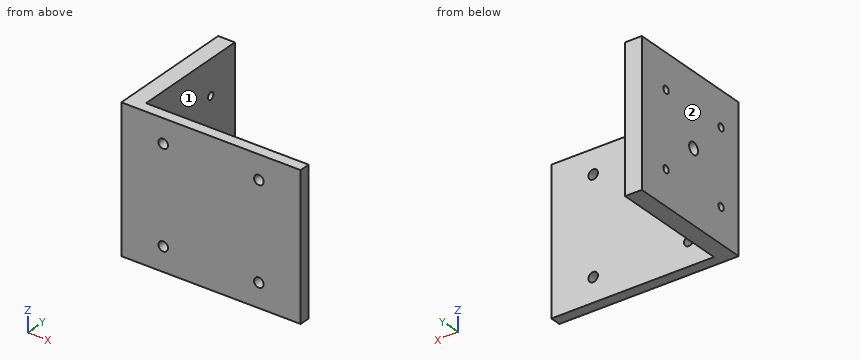
```python
from build123d import *

# Parameters (mm, degrees)
SKETCH1_W           = 75
SKETCH1_H           = 60
BOSS_EXTRUDE1_DEPTH = 4.5
SKETCH2_W           = 7
SKETCH2_H           = 60
BOSS_EXTRUDE2_DEPTH = 50
SKETCH3_R           = 1.5
SKETCH3_R_2         = 2.5
CUT_EXTRUDE1_DEPTH  = 10
SKETCH6_R           = 2
CUT_EXTRUDE2_DEPTH  = 10


with BuildPart() as part:
    # Sketch1 → Boss-Extrude1 (new body)
    with BuildSketch(Plane(origin=(0, 0, 0), x_dir=(1, 0, 0), z_dir=(0, 1, 0))):
        Rectangle(SKETCH1_W, SKETCH1_H)
    extrude(amount=BOSS_EXTRUDE1_DEPTH)

    # Sketch2 → Boss-Extrude2 (add)
    with BuildSketch(Plane(origin=(0, 4.5, 0), x_dir=(1, 0, 0), z_dir=(0, 1, 0))):
        with Locations((-34, 0)):
            Rectangle(SKETCH2_W, SKETCH2_H)
    extrude(amount=BOSS_EXTRUDE2_DEPTH)

    # Sketch3 → Cut-Extrude1 (cut)
    with BuildSketch(Plane.ZY.offset(37.5)):
        with Locations((-15.5, 40.9)):
            Circle(SKETCH3_R)
        with Locations((15.5, 40.9)):
            Circle(SKETCH3_R)
        with Locations((15.5, 9.9)):
            Circle(SKETCH3_R)
        with Locations((-15.5, 9.9)):
            Circle(SKETCH3_R)
        with Locations((0, 25.4)):
            Circle(SKETCH3_R_2)
    extrude(amount=-CUT_EXTRUDE1_DEPTH, mode=Mode.SUBTRACT)

    # Sketch6 → Cut-Extrude2 (cut)
    with BuildSketch(Plane(origin=(0, 4.5, 0), x_dir=(1, 0, 0), z_dir=(0, 1, 0))):
        with Locations(Location((20, 20, 0), (0, 0, 270))):
            Circle(SKETCH6_R)
        with Locations(Location((-20, 20, 0), (0, 0, 270))):
            Circle(SKETCH6_R)
        with Locations(Location((20, -20, 0), (0, 0, 270))):
            Circle(SKETCH6_R)
        with Locations(Location((-20, -20, 0), (0, 0, 270))):
            Circle(SKETCH6_R)
    extrude(amount=-CUT_EXTRUDE2_DEPTH, mode=Mode.SUBTRACT)


solid = part.part
```
Model file for the job. Use its own axes, mm. Face numbers are marked on the shaded views. A direction names the side the tool comes from. Round coordinates to 2 decimals unless told otherwise and drop trailing zeros. Write each loop counter-clockwise with the first axis right and the second up, starting at its lowest first coordinate (ties: lowest second). Pieces come first, ordered by that corner, then holes. Notation, with made-up numbers: M 54.25,-24 L 111.25,-24 A21 cw 111.25,-5 Z; hole C -11.75,49.25 d1. An arc over 180 degrees is marked long. Put each result on its own line as item: value.
Item 1: Tool access for the marked faces 1 and 2: list every direction of +Z, -Z, +X, -X, +Y, -Y with a clear straight run to the whole face (end or side of a thin tool).
Responses:
face 1: +Z, -Z, +X, +Y
face 2: +Z, -Z, -X, +Y, -Y
Item 2: Cut at B-B (x = -20). List the corners of the cut face in (y, z).
Responses:
outline: M 0,-30 L 4.5,-30 L 4.5,-22 L 0,-22 Z; M 0,-18 L 4.5,-18 L 4.5,18 L 0,18 Z; M 0,22 L 4.5,22 L 4.5,30 L 0,30 Z
Item 3: Cut at D-D (y = 9.9). List the corners of the cut face in (x, z), and give its area (3 significant figures).
Responses:
outline: M -37.5,-30 L -30.5,-30 L -30.5,-17 L -37.5,-17 Z; M -37.5,-14 L -30.5,-14 L -30.5,14 L -37.5,14 Z; M -37.5,17 L -30.5,17 L -30.5,30 L -37.5,30 Z
area: 378 mm²
Item 4: Cut at C-C (z = 0). List the corners of the cut face in (x, y).
Responses:
outline: M -37.5,0 L 37.5,0 L 37.5,4.5 L -30.5,4.5 L -30.5,22.9 L -37.5,22.9 Z; M -37.5,27.9 L -30.5,27.9 L -30.5,54.5 L -37.5,54.5 Z
Item 5: Flat gauge pins, fed straight in: P1, Ø3.5, axis at y = 40.9, z = -15.5, coming from the +X side; P2, Ø2.5, axis at y = 9.9, z = -15.5, coming from the -X side; P3, Ø12, axis at x = 22, z = 5.5, coming from the +Y side. Where does each tip first touch, or does it go through?
Responses:
P1: x = -30.5
P2: through
P3: y = 4.5
Item 6: Cut at A-A (z = 15.5). List the corners of the cut face in (x, y), and give its area (4 significant figures).
Responses:
outline: M -37.5,0 L 37.5,0 L 37.5,4.5 L -30.5,4.5 L -30.5,8.4 L -37.5,8.4 Z; M -37.5,11.4 L -30.5,11.4 L -30.5,39.4 L -37.5,39.4 Z; M -37.5,42.4 L -30.5,42.4 L -30.5,54.5 L -37.5,54.5 Z
area: 645.5 mm²
Item 7: Probe L1, parallel to X at y = 1, z = -20; L2, parallel to X at y = 34, z = 23.5; L3, parallel to Y at x = 13, z = 6. List the from-to ranges inside material, lowest first. Write a range as from..to.
Responses:
L1: -37.5..-22, -18..18, 22..37.5
L2: -37.5..-30.5
L3: 0..4.5
